```python
from build123d import *

# Parameters (mm, degrees)
SKETCH1_W               = 381
SKETCH1_H               = 381
SKETCH1_R               = 4.064
SKETCH1_R_2             = 2.54
SKETCH1_R_3             = 6.223
SKETCH1_R_4             = 2.5796875
SKETCH1_R_5             = 1.5875
BOSS_EXTRUDE1_DEPTH     = 6.35
F_3_8_24_TAPPED_HOLE2_D = 8.4328


with BuildPart() as part:
    # Sketch1 → Boss-Extrude1 (new body)
    with BuildSketch(Plane.XY):
        with Locations((0, 190.5)):
            Rectangle(SKETCH1_W, SKETCH1_H)
        with Locations((76.2, 273.05)):
            Circle(SKETCH1_R, mode=Mode.SUBTRACT)
        with Locations((44.45, 241.3)):
            Circle(SKETCH1_R_2, mode=Mode.SUBTRACT)
        with Locations((88.9, 95.25)):
            Circle(SKETCH1_R_3, mode=Mode.SUBTRACT)
        with Locations(Location((-165.1, 25.4, 0), (0, 0, 180))):
            Circle(SKETCH1_R_2, mode=Mode.SUBTRACT)
        with Locations((101.2, 298.05)):
            Circle(SKETCH1_R_2, mode=Mode.SUBTRACT)
        with Locations((158.75, 190.5)):
            Circle(SKETCH1_R_2, mode=Mode.SUBTRACT)
        with Locations((101.2, 248.05)):
            Circle(SKETCH1_R_2, mode=Mode.SUBTRACT)
        with Locations((165.1, 25.4)):
            Circle(SKETCH1_R_2, mode=Mode.SUBTRACT)
        with Locations(Location((-88.9, 95.25, 0), (0, 0, 180))):
            Circle(SKETCH1_R_3, mode=Mode.SUBTRACT)
        with Locations(Location((-146.05, 190.5, 0), (0, 0, 180))):
            Circle(SKETCH1_R_2, mode=Mode.SUBTRACT)
        with Locations((51.2, 298.05)):
            Circle(SKETCH1_R_2, mode=Mode.SUBTRACT)
        with Locations((-25.4, 301.365)):
            Circle(SKETCH1_R_4, mode=Mode.SUBTRACT)
        with Locations((25.4, 301.365)):
            Circle(SKETCH1_R_4, mode=Mode.SUBTRACT)
        with Locations(Location((-44.45, 241.3, 0), (0, 0, 180))):
            Circle(SKETCH1_R_2, mode=Mode.SUBTRACT)
        with Locations(Location((-76.2, 273.05, 0), (0, 0, 180))):
            Circle(SKETCH1_R, mode=Mode.SUBTRACT)
        with Locations((-95.25, 316.23)):
            Circle(SKETCH1_R_5, mode=Mode.SUBTRACT)
    extrude(amount=BOSS_EXTRUDE1_DEPTH)

    # 3/8-24 Tapped Hole2 (through all)
    with Locations(Plane.XY.offset(6.35)):
        with Locations((-146.05, 279.4)):
            Hole(F_3_8_24_TAPPED_HOLE2_D / 2)


solid = part.part
```
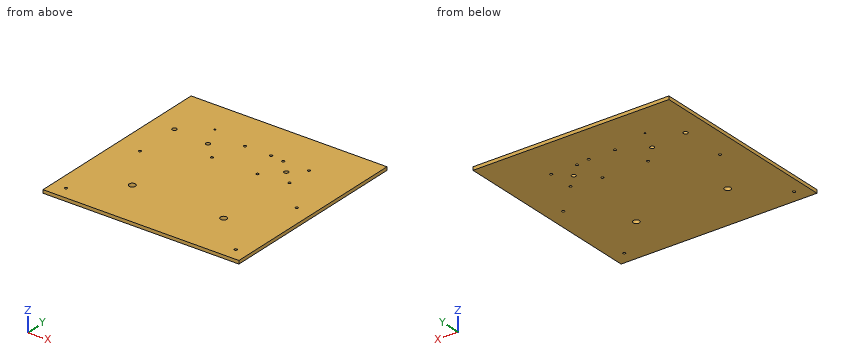
The listing builds one solid part. Answer for the finished solid, in the listing's coordinates (mm). Coordinates: 2 decimals unless noted, no trailing zeros. Write each loop counter-clockwise with the first axis right and the second up, starting at its lowest first coordinate (ties: lowest second). Pieces come first, ordered by that corner, then holes. Notation, with made-up numbers: M 67.5,9 L 101.5,9 A28 cw 101.5,43 Z; hole C 89,6.5 d6. An arc over 180 degrees is marked long. Use a Markdown table: item, result. Add a question column.
1. Straight lines are drawn through the part: line 1 along Y through (x, z) = (-146.05, 3.25); line 2 along X through (y, z) = (279.4, 2.75); line 3 along Y through (x, z) = (-95.25, 2.75). For each, find the intervals that lie inside material, in ascending order. Write a range as [from, to].
2. Section A-A (y = 95.25) is taken. Give the vertices of the cut face in (x, z).
3. Given P1, Ø8, axis at x = -44.45, y = 241.3, coming from the -Z side, flat-ended and moving along its own axis, determine where the tip first touches the part or whether it passes through.
Data:
| question | item | result |
|---|---|---|
| 1 | line 1 | y = [0, 187.96], [193.04, 275.18], [283.62, 381] |
| 1 | line 2 | x = [-190.5, -150.27], [-141.83, 190.5] |
| 1 | line 3 | y = [0, 314.64], [317.82, 381] |
| 2 | outline | M -190.5,0 L -95.12,0 L -95.12,6.35 L -190.5,6.35 Z; M -82.68,0 L 82.68,0 L 82.68,6.35 L -82.68,6.35 Z; M 95.12,0 L 190.5,0 L 190.5,6.35 L 95.12,6.35 Z |
| 3 | P1 | stops at z = 0 |
